Could you check a few things on this drawing? It's one solid part, dimensions in mm from its lowest x, y, z. Give positions to 0.01 mm unless a question says otherwise; leave off trailing zeros. Order: outer loops, then holes, each group sorted by start corner. A loop starts at its lowest first (then second) coordinate and runs counter-clockwise, first axis right, second up. Notation, with made-up numbers: (13.25, 33) - (54.25, 33) arc R24 cw to (54.25, 43) - close; hole circle Ø4 at (5.5, 34). An arc over 180 degrees is marked (long way). One line per question, with ' | ' between items. Start each with the question number.
1. Imagine slicing it at B-B (z = 13.5). Please give me the cut outline in (x, y), and give its area (3 significant figures).
2. I need wall thicknesses on probe 1 along Z at (x, y) = (2.25, 2); probe 2 along Y at (x, z) = (4, 15); probe 3 along X at (y, z) = (8.75, 8) (1 decimal). Which ranges of each line are inside material? Lowest first, please. Write a range as from..to.
3. Imagine slicing it at C-C (x = 4). Please give me the cut outline in (y, z).
4. Imagine slicing it at A-A (y = 7). Please give me the cut outline in (x, z).
5. For P1, Ø3, axis at x = 9.5, z = 18.5, coming from the +Y side; P2, Ø1, axis at x = 10, z = 7, coming from the -Y side; P3, Ø2.5, axis at x = 12, y = 8, coming from the +Z side; P4, Ø3, axis at x = 9.5, y = 8.5, coming from the +Z side, each with a flat end and sliding along its axis, tell me the tip position at first contact or that it passes through.
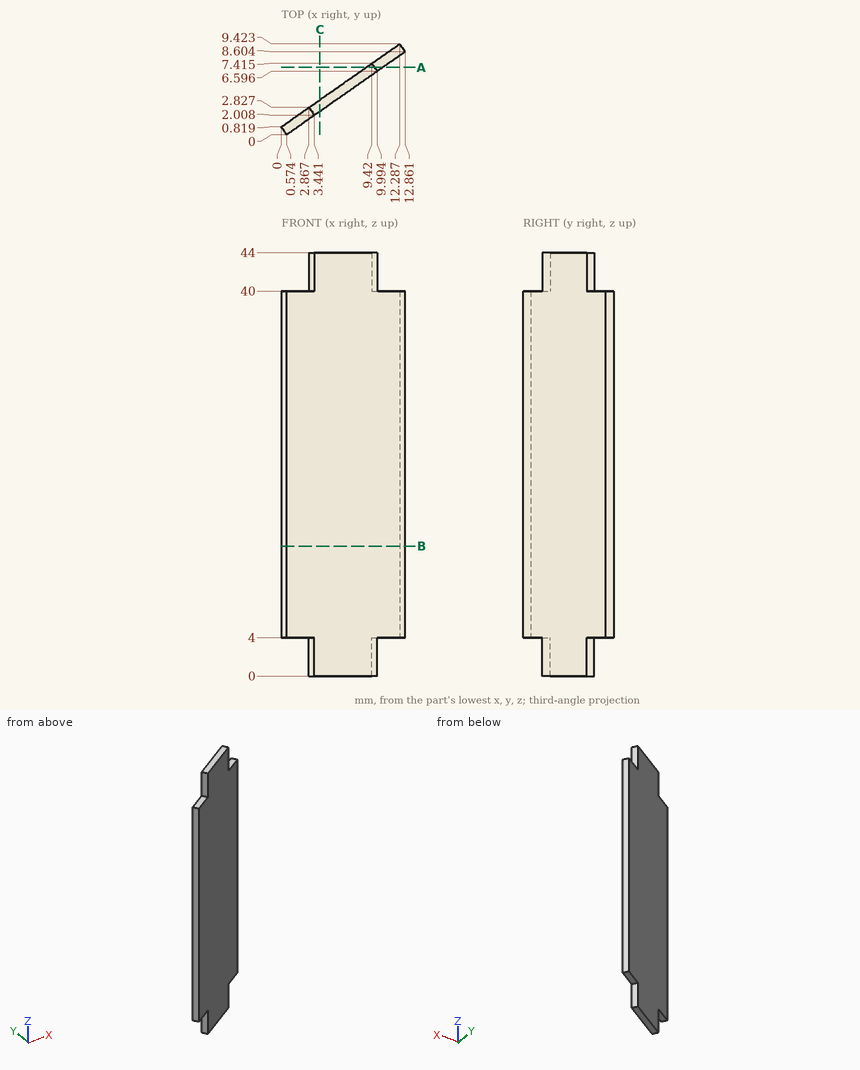
Results found:
1) outline: (0, 0.82) - (0.57, 0) - (12.86, 8.6) - (12.29, 9.42) - close | area: 15.0 mm2
2) probe 1: z = 4..40 | probe 2: y = 2.4..3.62 | probe 3: x = 11.3..12.8
3) outline: (2.4, 0) - (3.62, 0) - (3.62, 44) - (2.4, 44) - close
4) outline: (8.83, 0) - (9.71, 0) - (9.71, 4) - (10.57, 4) - (10.57, 40) - (9.71, 40) - (9.71, 44) - (8.83, 44) - close
5) P1: stops at y = 8.52 | P2: stops at y = 6.25 | P3: stops at z = 40 | P4: stops at z = 44
